The figure shows three views and two pictorial views of one solid part (mm, origin at its lowest corner). Answer the questions. Give positions to 0.01 mm unless a question says otherwise; leave off trailing zeros. Write each loop counter-clockwise with the first axis right and the second up, starting at its lowest first coordinate (ties: lowest second). Pieces come first, ordered by that corner, then holes. Notation, with made-up numbers: M 39,-13.5 L 74,-13.5 A19 cw 74,1.5 Z; hole C 49,-29.5 d8. An arc over 180 degrees is marked long. Return JSON: item names as keys, results as strings.
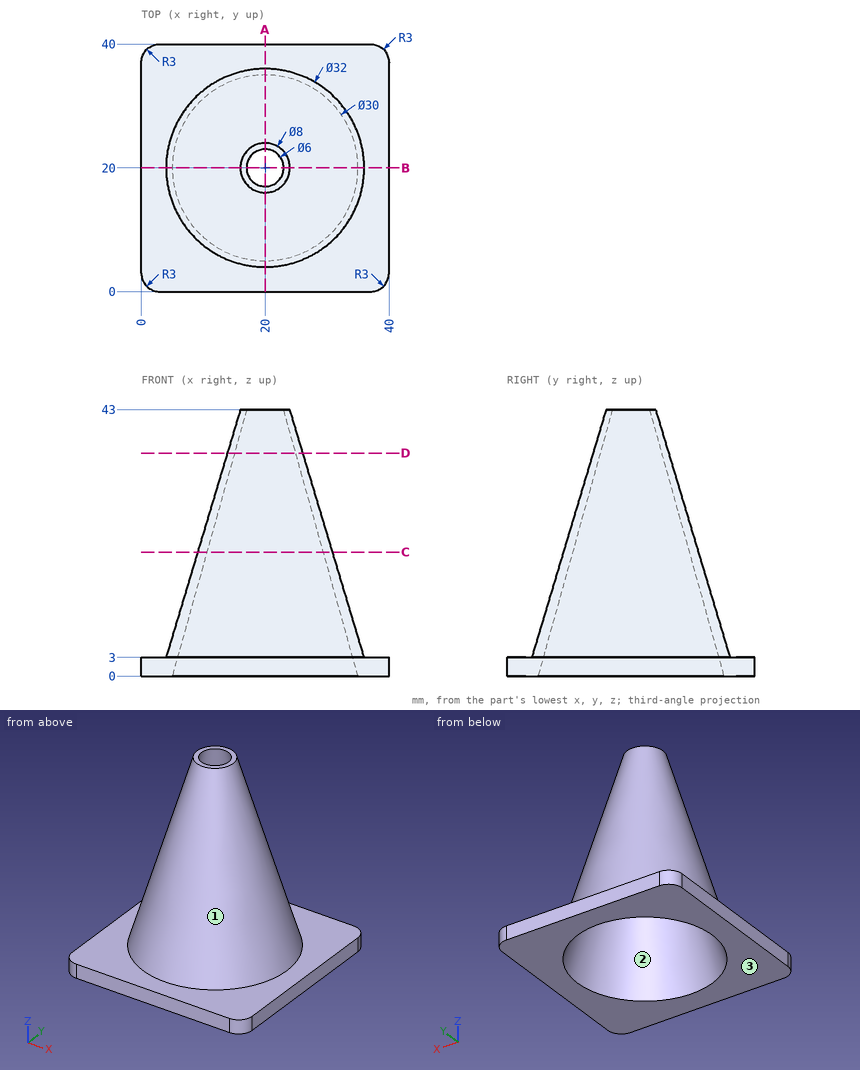
Item 1: Determine the mould class of the marked faces 1, 2 and 3 for opening direction Y: +Y half, -Y half, draft (parallel to the pull), parting line (faces both ways), or undercut.
Geometry results:
{"face 1": "parting line", "face 2": "undercut", "face 3": "draft"}
Item 2: A cutting plane is placed at D-D, the plane z = 36. Write down the section's boundary in (x, y), plus the area to 3 significant figures.
Geometry results:
{"outline": "C 20,20 d12.2; hole C 20,20 d9.91", "area": "39.8 mm2"}
Item 3: Given pin 1 Ø2 at (y, z) = (26, 30) entering from -X; pin 2 Ø8 at (x, z) = (29.5, 14.5) entering from +Y; pin 3 Ø10 at (y, z) = (36, 16) entering from -X, each flat-ended and moving along its own axis, determine where each tip first touches the part or whether it passes through.
Geometry results:
{"pin 1": "stops at x = 13.8", "pin 2": "stops at y = 31.69", "pin 3": "stops at x = 14.4"}
Item 4: A cutting plane is placed at A-A, the plane x = 20. Write down the section's boundary in (y, z).
Geometry results:
{"outline": "M 0,0 L 5,0 L 17,43 L 16,43 L 4,3 L 0,3 Z; M 23,43 L 35,0 L 40,0 L 40,3 L 36,3 L 24,43 Z"}
Item 5: Find the intervals of material crossed by line 1 (Z direction, x = 36.5, y = 30.5); line 2 (X direction, y = 20, z = 6); line 3 (Y direction, x = 12.5, z = 17), in increasing order.
Geometry results:
{"line 1": "z = 0 to 3", "line 2": "x = 4.9 to 6.67, 33.33 to 35.1", "line 3": "y = 10.89 to 13, 27 to 29.11"}
Item 6: A cutting plane is placed at C-C, the plane z = 20. Write down the section's boundary in (x, y).
Geometry results:
{"outline": "C 20,20 d21.8; hole C 20,20 d18.84"}
